Part model, mm, in its own coordinate system. A direction names the side the tool comes from. Give positions to 0.01 mm unless a question says otherwise; leave off trailing zeros. Write each loop counter-clockwise with the first axis right and the second up, starting at its lowest first coordinate (ties: lowest second). Pieces come first, ordered by that corner, then holes. Notation, with made-up numbers: M -30.75,43 L 18.25,43 A10 ccw 18.25,49 Z; hole C 74,-20 d6. An arc over 180 degrees is marked long. Use CSV: the item, a comma, the result in double quotes. Start each with the question number.
1. Band-saw the part on B-B, the plane z = 16.5. List the corners of the cut face in (x, y).
2. Drill centre lines: line 1 along X through (y, z) = (-7.25, 17.25); line 2 along Y through (x, z) = (-19.5, 15.25); line 3 along Y through (x, z) = (-28.25, 14.5). Where is each one in solid material? Low to high. Write a range as from..to.
3. Mould opens along X. For faces 1 (the face through (-27, -6, 17.747)), 2 (the face through (-24.428, -2, 17)), 3 (the face through (-23.778, -6, 17)), 4 (the face through (-30.103, -3, 13)) say: pulls with the +X half, pulls with the -X half, needs draft (parallel to the pull), parting line crosses it, or undercut.
4. 3-axis set-ups, long thin cutter, end or side, ignore diameter. For faces 5 (the face through (-21, -2, 17.747)), 6 (the face through (-25.52, -4.04, 15.45)), 7 (the face through (-24.428, -6, 17)): which of +Z, -Z, +X, -X, +Y, -Y reach the whole face in a straight line?
5. Band-saw the part on C-C, the plane y = -1. List the corners of the cut face in (x, z) (3 decimals), then the cut area to 3 significant figures.
6. Band-saw the part on A-A, the plane x = -27.25. List the corners of the cut face in (y, z), then the cut area to 3 significant figures.
7. Band-saw the part on D-D, the plane x = -22.5. Count the separate pieces of the cut face and the enclosed holes in it, then the cut area to 3 significant figures.
from build123d import *

# Parameters (mm, degrees)
F1_DEPTH = 8
F2_SIZE  = 0.25
F4_W     = 17.8603331085
F4_H     = 0.65
F5_DEPTH = 6.5


with BuildPart() as f1:
    # F0 (on Front) → F1 (new body)
    with BuildSketch(Plane.XZ):
        with BuildLine():
            Line((-24.4284769839, 17.7468117975), (-30.1034769839, 17.7468117975))
            Line((-30.1034769839, 17.7468117975), (-30.1034769839, 7.7468117975))
            Line((-30.1034769839, 7.7468117975), (-18.1034769839, 7.7468117975))
            Line((-18.1034769839, 7.7468117975), (-18.1034769839, 17.7468117975))
            Line((-18.1034769839, 17.7468117975), (-23.7784769839, 17.7468117975))
            Line((-23.7784769839, 17.7468117975), (-23.7784769839, 15.5934303288))
            ThreePointArc((-23.7784769839, 15.5934303288), (-22.6673363223, 14.9522681427), (-22.2284769839, 13.7468117975))
            ThreePointArc((-22.2284769839, 13.7468117975), (-25.308933329, 12.3106711359), (-24.4284769839, 15.5934303288))
            Line((-24.4284769839, 15.5934303288), (-24.4284769839, 17.7468117975))
        make_face()
    extrude(amount=F1_DEPTH)

    # F2
    f2_edges = [f1.edges().sort_by_distance(p)[0] for p in [
        (-24.103477, 0, 11.871812),
        (-24.103477, -8, 11.871812),
    ]]
    chamfer(f2_edges, length=F2_SIZE)

    # F4 (on face) → F5 (cut)
    with BuildSketch(Plane(origin=(0, -2.2654882704, 18.4509213023), x_dir=(1, 0, 0), z_dir=(0, 0.1218693434, -0.9925461516))):
        with Locations((-24.4247596711, 2.4525769118)):
            Rectangle(F4_W, F4_H)
    extrude(amount=F5_DEPTH, mode=Mode.SUBTRACT)


solid = f1.part
Output:
1,outline,"M -30.1,-8 L -24.43,-8 L -24.43,-4.82 L -30.1,-4.82 Z; M -30.1,-4.17 L -24.43,-4.17 L -24.43,0 L -30.1,0 Z; M -23.78,-8 L -18.1,-8 L -18.1,-4.82 L -23.78,-4.82 Z; M -23.78,-4.17 L -18.1,-4.17 L -18.1,0 L -23.78,0 Z"
2,line 1,"x = -30.1..-24.43, -23.78..-18.1"
2,line 2,"y = -8..-4.67, -4.02..0"
2,line 3,"y = -8..-4.58, -3.92..0"
3,face 1,"needs draft"
3,face 2,"undercut"
3,face 3,"undercut"
3,face 4,"pulls with the -X half"
4,face 5,"+Z, +X, -X, +Y, -Y"
4,face 6,"+X, -X"
4,face 7,"+Z, +Y, -Y"
5,outline,"M -30.103,7.747 L -18.103,7.747 L -18.103,17.747 L -23.778,17.747 L -23.778,15.593 A1.875 cw long -24.428,15.593 L -24.428,17.747 L -30.103,17.747 Z"
5,area,"108 mm²"
6,outline,"M -8,7.75 L 0,7.75 L 0,17.75 L -4.32,17.75 L -3.59,11.74 L -4.23,11.66 L -4.98,17.75 L -8,17.75 Z"
6,area,"76.0 mm²"
7,separate pieces,"3"
7,enclosed holes,"0"
7,area,"61.5 mm²"
